Could you check a few things on this model? Use its own coordinates, in mm. A direction names the side the tool comes from. Round coordinates to 2 decimals unless told otherwise and drop trailing zeros. Write each loop counter-clockwise with the first axis right and the second up, starting at its lowest first coordinate (ties: lowest second). Pieces come first, ordered by that corner, then holes. Notation, with made-up numbers: (-4, 86) -> (36, 86) arc R25 ccw to (36, 113) -> close; hole circle Ø2 at (10, 56). An arc over 180 degrees is marked (long way). Answer as CSV lines item,"result". Start each with the question number.
Q1. Will these pins go through, and if not, where does the flat tip stop? pin 1 Ø1.2 at (y, z) = (8, -11.5) entering from +X; pin 2 Ø4 at (x, z) = (4.5, -5) entering from +Y; pin 3 Ø3 at (y, z) = (5.5, -9.5) entering from -X; pin 4 Ø4.5 at (y, z) = (6.5, -13) entering from -X.
Q2. Imagine slicing it at A-A on y = 8.5. Please give me the cut outline in (x, z).
Q3. If I drill on line 1 (Z direction, x = -0.5, y = 5); line 2 (Z direction, x = -3.5, y = 7.25); line 3 (X direction, y = 1.25, z = 3.5), over which ranges is the centre line in solid material (lowest first)? Write a range as [from, to].
Q4. Imagine slicing it at D-D on z = -3. Please give me the cut outline in (x, y).
Q5. If we mould it in two halves opening along Y, with no side actions, what happens to faces 1 (the flat face through (0, 4, -14.5)), 2 (the flat face through (0, 10, -15)), 3 (the flat face through (1.5, 7, 13))? For each: pulls with the +Y half, pulls with the -Y half, needs draft (parallel to the pull), parting line crosses it, or undercut.
Q6. Imagine slicing it at C-C on z = -13.5. Please give me the cut outline in (x, y).
Q7. For faces 4 (the flat face through (0, 8, -12.5)), 5 (the flat face through (0, 4.939, 12)), 6 (the flat face through (-1.5, 7, -13)), which set-ups out of +Z, -Z, +X, -X, +Y, -Y let a thin tool reach every point of the face, with its end or its side?
from build123d import *

# Parameters (mm, degrees)
SKETCH1_W           = 34
SKETCH1_H           = 32
BOSS_EXTRUDE1_DEPTH = 2
SKETCH4_W           = 4
SKETCH4_H           = 8
BOSS_EXTRUDE2_DEPTH = 1.5
BOSS_EXTRUDE5_DEPTH = 1.5
MIRROR1_START       = -4
MIRROR1_OUTLINE_W   = 8
MIRROR1_OUTLINE_H   = 1.5
MIRROR1_DEPTH       = 8
MIRROR1_START_2     = -1.5
MIRROR1_2_DEPTH     = 3
SKETCH7_W           = 4.713008878
SKETCH7_H           = 21.4981103
CUT_EXTRUDE1_DEPTH  = 7.5


# Read off the part's stored shape, not the designer's step: Mirror1
with BuildPart() as part:
    # Sketch1 → Boss-Extrude1 (new body)
    with BuildSketch(Plane(origin=(0, 0, 0), x_dir=(1, 0, 0), z_dir=(0, 1, 0))):
        Rectangle(SKETCH1_W, SKETCH1_H)
    extrude(amount=BOSS_EXTRUDE1_DEPTH)

    # Sketch4 → Boss-Extrude2 (add)
    with BuildSketch(Plane(origin=(0, 0, -16), x_dir=(-1, 0, 0), z_dir=(0, 0, -1))):
        with Locations((2, 6)):
            Rectangle(SKETCH4_W, SKETCH4_H)
    extrude(amount=-BOSS_EXTRUDE2_DEPTH)

    # Sketch5 → Boss-Extrude5 (add)
    with BuildSketch(Plane(origin=(0, 0, 0), x_dir=(0, 0, -1), z_dir=(1, 0, 0))):
        Polygon((14.5, 10), (10.439339828, 5.939339828), (10.439339828, 4.939339828), (14.5, 4.939339828), (14.5, 2), (16, 2), (16, 10), align=None)
    extrude(amount=-BOSS_EXTRUDE5_DEPTH)

    # Mirror1 outline → Mirror1 (add)
    with BuildSketch(Plane.YZ.offset(MIRROR1_START)):
        with Locations((6, 15.25)):
            Rectangle(MIRROR1_OUTLINE_W, MIRROR1_OUTLINE_H)
        with Locations((6, -15.25)):
            Rectangle(MIRROR1_OUTLINE_W, MIRROR1_OUTLINE_H)
    extrude(amount=MIRROR1_DEPTH)

    # Mirror1 2 outline → Mirror1 2 (add)
    with BuildSketch(Plane.YZ.offset(MIRROR1_START_2)):
        Polygon((4.939339828, -14.5), (10, -14.5), (5.939339828, -10.439339828), (4.939339828, -10.439339828), align=None)
        Polygon((10, 14.5), (4.939339828, 14.5), (4.939339828, 10.439339828), (5.939339828, 10.439339828), align=None)
    extrude(amount=MIRROR1_2_DEPTH)

    # Sketch7 → Cut-Extrude1 (cut)
    with BuildSketch(Plane(origin=(0, 2, 0), x_dir=(1, 0, 0), z_dir=(0, 1, 0))):
        with Locations((-10.988574464, 5.211128947)):
            Rectangle(SKETCH7_W, SKETCH7_H)
    extrude(amount=-CUT_EXTRUDE1_DEPTH, mode=Mode.SUBTRACT)


solid = part.part
Checks:
1,pin 1,"through"
1,pin 2,"y = 2"
1,pin 3,"x = -1.5"
1,pin 4,"x = -4"
2,outline,"(-4, -16) -> (4, -16) -> (4, -14.5) -> (1.5, -14.5) -> (1.5, -13) -> (-1.5, -13) -> (-1.5, -14.5) -> (-4, -14.5) -> close; (-4, 14.5) -> (-1.5, 14.5) -> (-1.5, 13) -> (1.5, 13) -> (1.5, 14.5) -> (4, 14.5) -> (4, 16) -> (-4, 16) -> close"
3,line 1,"[-16, -10.44], [10.44, 16]"
3,line 2,"[-16, -14.5], [14.5, 16]"
3,line 3,"[-17, -13.35], [-8.63, 17]"
4,outline,"(-17, 0) -> (-13.35, 0) -> (-13.35, 2) -> (-17, 2) -> close; (-8.63, 0) -> (17, 0) -> (17, 2) -> (-8.63, 2) -> close"
5,face 1,"undercut"
5,face 2,"pulls with the +Y half"
5,face 3,"needs draft"
6,outline,"(-17, 0) -> (-13.35, 0) -> (-13.35, 2) -> (-17, 2) -> close; (-8.63, 0) -> (17, 0) -> (17, 2) -> (-8.63, 2) -> close; (-1.5, 4.94) -> (1.5, 4.94) -> (1.5, 9) -> (-1.5, 9) -> close"
7,face 4,"+X, -X, +Y"
7,face 5,"+X, -X"
7,face 6,"-X, +Y"
